from build123d import *

# Parameters (mm, degrees)
F0_R     = 6.425
F1_DEPTH = 12
F2_R     = 1.5
F3_DEPTH = 12.5
F5_DEPTH = 1.75
F6_W     = 3.5
F6_H     = 0.3499913151
F6_W_2   = 2.4
F6_H_2   = 1.6
F6_H_3   = 3
F6_H_4   = 1.8378814235
F7_DEPTH = 12.5


with BuildPart() as f1:
    # F0 (on Top) → F1 (new body)
    with BuildSketch(Plane.XY):
        Circle(F0_R)
    extrude(amount=-F1_DEPTH)

    # F2 (on Front) → F3 (cut, symmetric)
    with BuildSketch(Plane.XZ):
        with Locations((0, -8.6621185765)):
            Circle(F2_R)
    extrude(amount=F3_DEPTH, both=True, mode=Mode.SUBTRACT)

    # F4 (on Front) → F5 (cut, symmetric)
    with BuildSketch(Plane.XZ):
        with BuildLine():
            Line((6.425, -12), (2.7726078369, -6.7377301586))
            ThreePointArc((2.7726078369, -6.7377301586), (0, -5.2871185765), (-2.7726078369, -6.7377301586))
            Line((-2.7726078369, -6.7377301586), (-6.425, -12))
            Line((-6.425, -12), (6.425, -12))
        make_face()
    extrude(amount=F5_DEPTH, both=True, mode=Mode.SUBTRACT)

    # F6 (on Right) → F7 (cut, symmetric)
    with BuildSketch(Plane.YZ):
        with Locations((0, -11.8250043425)):
            Rectangle(F6_W, F6_H)
        with Locations((-5.225, -6.3621185765)):
            Rectangle(F6_W_2, F6_H_2)
        with Locations((-5.225, -8.6621185765)):
            Rectangle(F6_W_2, F6_H_3)
        with Locations((-5.225, -11.0810592882)):
            Rectangle(F6_W_2, F6_H_4)
    extrude(amount=F7_DEPTH, both=True, mode=Mode.SUBTRACT)


solid = f1.part
CAD build for the part. Positions are in the model's coordinates, mm. A direction names the side the tool comes from. Coordinates: 2 decimals unless noted, no trailing zeros. Loops run counter-clockwise (first coordinate to the right, second up) from the corner with the lowest first, then second, coordinate; pieces in that order, holes last. Notation, with made-up numbers: (14, 73.5) - (37, 73.5) arc R30 cw to (37, 107.5) - close; hole circle Ø4 at (2.5, 15.25). An arc over 180 degrees is marked (long way). Use one line per item in the form item = value. Start each with the question number.
1) Band-saw the part on D-D (y = -2.5). Give the cut face in (x, z), and give its area (3 significant figures).
2) Flat gauge pins, fed straight in: pin 1 (3 mm diameter, centred on x = 1.5, z = -10, fed in from -Y) (3 decimals); pin 2 (4 mm diameter, centred on y = 3, z = -6.5, fed in from -X); pin 3 (1.8 mm diameter, centred on x = 0, z = -8.66, fed in from +Y) (3 decimals); pin 4 (4 mm diameter, centred on x = -2.5, z = -5, fed in from -Y). Where does each tip first touch, or does it go through?
3) Band-saw the part on A-A (x = 0). Give the cut face in (y, z) (3 decimals).
4) Band-saw the part on C-C (z = -9.5). Give the cut face in (x, y) (3 decimals), and give its area (3 significant figures).
5) Tool access for faces 4 (the face through (0, -5, -5.562)), 5 (the face through (-0.325, 4.057, -10.126)), 6 (the face through (0, -1.75, -11)): list every direction of +Z, -Z, +X, -X, +Y, -Y with a clear straight run to the whole face (end or side of a thin tool).
6) Band-saw the part on B-B (y = 0). Give the cut face in (x, z) (3 decimals).
7) Drill centre lines: L1, parallel to Z at x = 0, y = 3.8; L2, parallel to X at y = 1.5, z = -9.25; L3, parallel to Y at x = 0.25, z = -5.5. Where is each one in solid material? Low to high. Write a range as from..to.
8) Two-plate mould, pull along X, no slides. Class faces 1 (the face through (0, -3, -12)), 2 (the face through (-0.325, -2.903, -10.126)), 3 (the face through (-0.84, 6.37, -5.92)): +X half, -X half, draft (parallel to the pull), parting line (faces both ways), or undercut.
Check values:
q1.outline = (-5.92, -12) - (5.92, -12) - (5.92, 0) - (-5.92, 0) - close; hole circle Ø3 at (0, -8.66)
q1.area = 135 mm2
q2.pin_1 = -4.025
q2.pin_2 = -6.35
q2.pin_3 = through
q2.pin_4 = -6.41
q3.outline = (-6.425, -5.562) - (-4.025, -5.562) - (-4.025, -7.162) - (-1.75, -7.162) - (-1.75, -5.287) - (1.75, -5.287) - (1.75, -7.162) - (6.425, -7.162) - (6.425, 0) - (-6.425, 0) - close; (-4.025, -12) - (-1.75, -12) - (-1.75, -10.162) - (-4.025, -10.162) - close; (1.75, -12) - (6.425, -12) - (6.425, -10.162) - (1.75, -10.162) - close
q4.outline = (-5.008, -4.025) - (-1.244, -4.025) - (-1.244, -1.75) - (-4.69, -1.75) - (-4.69, 1.75) - (-1.244, 1.75) - (-1.244, 6.303) arc R6.425 ccw to start; (1.244, -4.025) - (5.008, -4.025) arc R6.425 ccw to (1.244, 6.303) - (1.244, 1.75) - (4.69, 1.75) - (4.69, -1.75) - (1.244, -1.75) - close
q4.area = 62.9 mm2
q5.face_4 = -Z, +X, -X, -Y
q5.face_5 = +Y, -Y
q5.face_6 = -Z
q6.outline = (-6.425, -11.65) - (-6.182, -11.65) - (-2.773, -6.738) arc R3.375 cw to (2.773, -6.738) - (6.182, -11.65) - (6.425, -11.65) - (6.425, 0) - (-6.425, 0) - close
q7.L1 = -12..-10.16, -7.16..0
q7.L2 = -6.25..-4.52, 4.52..6.25
q7.L3 = -6.42..-1.75, 1.75..6.42
q8.face_1 = draft
q8.face_2 = undercut
q8.face_3 = parting line
